```python
from build123d import *

# Parameters (mm, degrees)
SKETCH_W        = 130
SKETCH_H        = 300
PAD_DEPTH       = 15
SKETCH001_R     = 2.1
POCKET_DEPTH    = 15.001
SKETCH002_R     = 3
SKETCH002_R_2   = 4
POCKET001_DEPTH = 15.001


with BuildPart() as part:
    # Sketch → Pad (new body)
    with BuildSketch(Plane.XZ):
        with Locations((65, 150)):
            Rectangle(SKETCH_W, SKETCH_H)
    extrude(amount=PAD_DEPTH)

    # Sketch001 (on Face6 of Pad) → Pocket (cut, through all)
    with BuildSketch(Plane.XZ.offset(15)):
        with Locations((5, 280)):
            Circle(SKETCH001_R)
        with Locations((41, 280)):
            Circle(SKETCH001_R)
        with Locations((5, 248)):
            Circle(SKETCH001_R)
        with Locations((41, 248)):
            Circle(SKETCH001_R)
        with Locations((90, 280)):
            Circle(SKETCH001_R)
        with Locations((126, 280)):
            Circle(SKETCH001_R)
        with Locations((90, 248)):
            Circle(SKETCH001_R)
        with Locations((126, 248)):
            Circle(SKETCH001_R)
        with Locations((5, 90)):
            Circle(SKETCH001_R)
        with Locations((41, 90)):
            Circle(SKETCH001_R)
        with Locations((5, 58)):
            Circle(SKETCH001_R)
        with Locations((41, 58)):
            Circle(SKETCH001_R)
        with Locations((90, 90)):
            Circle(SKETCH001_R)
        with Locations((126, 90)):
            Circle(SKETCH001_R)
        with Locations((90, 58)):
            Circle(SKETCH001_R)
        with Locations((126, 58)):
            Circle(SKETCH001_R)
    extrude(amount=-POCKET_DEPTH, mode=Mode.SUBTRACT)

    # Sketch002 (on Face5 of Pocket) → Pocket001 (cut, through all)
    with BuildSketch(Plane.XZ.offset(15)):
        with Locations((9, 100)):
            Circle(SKETCH002_R)
        with Locations((121, 100)):
            Circle(SKETCH002_R)
        with Locations((65, 175)):
            Circle(SKETCH002_R_2)
        with Locations((65, 100)):
            Circle(SKETCH002_R_2)
        with Locations((19.127486, 132.12028)):
            Circle(SKETCH002_R)
        with Locations((110.872514, 67.87972)):
            Circle(SKETCH002_R)
        with Locations((19.127486, 67.87972)):
            Circle(SKETCH002_R)
        with Locations((110.872514, 132.12028)):
            Circle(SKETCH002_R)
    extrude(amount=-POCKET001_DEPTH, mode=Mode.SUBTRACT)


solid = part.part
```
For this review, take the finished solid that the model builds, in its own axes (mm). Coordinates: 2 decimals unless noted, no trailing zeros. Write each loop counter-clockwise with the first axis right and the second up, starting at its lowest first coordinate (ties: lowest second). Pieces come first, ordered by that corner, then holes. Notation, with made-up numbers: (-10.75, 28.5) -> (30.25, 28.5) arc R18 ccw to (30.25, 55.5) -> close; hole circle Ø4 at (-10.75, 73). An arc over 180 degrees is marked (long way). Put each result on its own line as item: value.
Q1. Wall thickness on L1, parallel to Z at x = 90, y = -11.5; L2, parallel to Z at x = 64.5, y = -9; L3, parallel to X at y = -6, z = 280: over which ranges is each line inside the solid? List them lowest first.
From the geometry:
L1: z = 0 to 55.9, 60.1 to 87.9, 92.1 to 245.9, 250.1 to 277.9, 282.1 to 300
L2: z = 0 to 96.03, 103.97 to 171.03, 178.97 to 300
L3: x = 0 to 2.9, 7.1 to 38.9, 43.1 to 87.9, 92.1 to 123.9, 128.1 to 130
Q2. The part is to be moulded in two halves that separate along Z. For faces 1 (the cylindrical face through (122.384, -7.605, 97.338)), 2 (the flat face through (64, -15, 152)), 3 (the flat face through (64, -7, 0)), 4 (the flat face through (64, -7, 300)), say which applies: +Z half, -Z half, draft (parallel to the pull), parting line (faces both ways), or undercut.
From the geometry:
face 1: undercut
face 2: draft
face 3: -Z half
face 4: +Z half
Q3. Take a section at C-C, the plane x = 65. State the section outline as (y, z) points.
From the geometry:
outline: (-15, 0) -> (0, 0) -> (0, 96) -> (-15, 96) -> close; (-15, 104) -> (0, 104) -> (0, 171) -> (-15, 171) -> close; (-15, 179) -> (0, 179) -> (0, 300) -> (-15, 300) -> close
Q4. Take a section at B-B, the plane z = 100. State the section outline as (x, y) points.
From the geometry:
outline: (0, -15) -> (6, -15) -> (6, 0) -> (0, 0) -> close; (12, -15) -> (61, -15) -> (61, 0) -> (12, 0) -> close; (69, -15) -> (118, -15) -> (118, 0) -> (69, 0) -> close; (124, -15) -> (130, -15) -> (130, 0) -> (124, 0) -> close
Q5. Take a section at A-A, the plane x = 121. State the section outline as (y, z) points, then the cut area to 3 significant figures.
From the geometry:
outline: (-15, 0) -> (0, 0) -> (0, 97) -> (-15, 97) -> close; (-15, 103) -> (0, 103) -> (0, 300) -> (-15, 300) -> close
area: 4,410 mm2
